```python
from build123d import *

# Parameters (mm, degrees)
SKETCH_1_R          = 18.5
SKETCH_1_R_2        = 15
EXTRUDE_1_DEPTH     = 4
SKETCH_2_R          = 17.8
SKETCH_2_R_2        = 15.7
CUT_EXTRUDE_1_DEPTH = 0.3


with BuildPart() as part:
    # 草图1 → 凸台-拉伸1 (new body)
    with BuildSketch(Plane(origin=(0, 0, 0), x_dir=(1, 0, 0), z_dir=(0, 1, 0))):
        with Locations(Location((0, 0, 0), (0, 0, 270))):
            Circle(SKETCH_1_R)
        with Locations(Location((0, 0, 0), (0, 0, 270))):
            Circle(SKETCH_1_R_2, mode=Mode.SUBTRACT)
    extrude(amount=EXTRUDE_1_DEPTH)

    # 草图2 → 切除-拉伸1 (cut)
    with BuildSketch(Plane(origin=(0, 4, 0), x_dir=(1, 0, 0), z_dir=(0, 1, 0))):
        with Locations(Location((0, 0, 0), (0, 0, 270))):
            Circle(SKETCH_2_R)
        with Locations(Location((0, 0, 0), (0, 0, 270))):
            Circle(SKETCH_2_R_2, mode=Mode.SUBTRACT)
    cut_extrude_1 = extrude(amount=-CUT_EXTRUDE_1_DEPTH, mode=Mode.SUBTRACT)

    # 镜向1: 切除-拉伸1 across plane
    add(cut_extrude_1.mirror(Plane.ZX.offset(2)), mode=Mode.SUBTRACT)


solid = part.part
```
Can you work these out from the model? Positions are in its coordinate system, mm. A direction names the side the tool comes from. Give positions to 0.01 mm unless a question says otherwise; leave off trailing zeros. Loops run counter-clockwise (first coordinate to the right, second up) from the corner with the lowest first, then second, coordinate; pieces in that order, holes last. Notation, with made-up numbers: M 13,35 L 62,35 A29 ccw 62,70 Z; hole C -4,30.5 d11. An arc over 180 degrees is marked long. One line per question, with ' | ' between items. Start each with the question number.
Q1. For faces 4 (the flat face through (15, 4, -10)), 5 (the flat face through (-16, 0.3, 0)), which set-ups out of +Z, -Z, +X, -X, +Y, -Y let a thin tool reach every point of the face, with its end or its side?
Q2. If we section it at A-A (z = -9.5): Please give me the cut outline in (x, y), plus the area to 3 significant figures.
Q3. For pin 1 Ø2 at (y, z) = (0.5, 3.5) entering from -X; pin 2 Ø1 at (y, z) = (2.5, 7) entering from +X, each with a flat end and sliding along its axis, tell me the tip position at first contact or that it passes through.
Q4. If we mould it in two halves opening along Z, with no side actions, what happens to faces 1 (the flat face through (-13, 4, 8)), 2 (the cylindrical face through (-7.086, 1.972, 17.089)), 3 (the flat face through (-16, 3.7, 0))? For each: +Z half, -Z half, draft (parallel to the pull), parting line (faces both ways), or undercut.
Q5. If I drill on line 1 (X direction, y = 0.1, z = 0); line 2 (X direction, y = 2.4, z = 0); line 3 (Z direction, x = -1, y = 0.25), over which ranges is the centre line in solid material (lowest first)? Write a range as from..to.
Q6. If we section it at B-B (x = 0): Please give me the cut outline in (y, z), plus the area to 3 significant figures.
Q7. If we section it at C-C (y = 2.35): Please give me the cut outline in (x, z), plus the area to 3 significant figures.
Computed:
1) face 4: +Z, -Z, +X, -X, +Y | face 5: -Y
2) outline: M -15.87,0 L -15.05,0 L -15.05,0.3 L -12.5,0.3 L -12.5,0 L -11.61,0 L -11.61,4 L -12.5,4 L -12.5,3.7 L -15.05,3.7 L -15.05,4 L -15.87,4 Z; M 11.61,0 L 12.5,0 L 12.5,0.3 L 15.05,0.3 L 15.05,0 L 15.87,0 L 15.87,4 L 15.05,4 L 15.05,3.7 L 12.5,3.7 L 12.5,4 L 11.61,4 Z | area: 31.1 mm²
3) pin 1: stops at x = -18.33 | pin 2: stops at x = 17.32
4) face 1: draft | face 2: parting line | face 3: undercut
5) line 1: x = -18.5..-17.8, -15.7..-15, 15..15.7, 17.8..18.5 | line 2: x = -18.5..-15, 15..18.5 | line 3: z = -18.47..-17.77, -15.67..-14.97, 14.97..15.67, 17.77..18.47
6) outline: M 0,-18.5 L 4,-18.5 L 4,-17.8 L 3.7,-17.8 L 3.7,-15.7 L 4,-15.7 L 4,-15 L 0,-15 L 0,-15.7 L 0.3,-15.7 L 0.3,-17.8 L 0,-17.8 Z; M 0,15 L 4,15 L 4,15.7 L 3.7,15.7 L 3.7,17.8 L 4,17.8 L 4,18.5 L 0,18.5 L 0,17.8 L 0.3,17.8 L 0.3,15.7 L 0,15.7 Z | area: 25.5 mm²
7) outline: C 0,0 d37; hole C 0,0 d30 | area: 368 mm²
